Verification items for the finished model (mm, model axes). Face numbers are marked on the shaded views. Round coordinates to 2 decimals unless told otherwise and drop trailing zeros. Write each loop counter-clockwise with the first axis right and the second up, starting at its lowest first coordinate (ties: lowest second). Pieces come first, ordered by that corner, then holes.
from build123d import *

# Parameters (mm, degrees)
ESBO_O1_R                = 3
RESSALTO_EXTRUS_O1_DEPTH = 5
FILETE1_R                = 6
RESSALTO_EXTRUS_O2_DEPTH = 5
ESBO_O3_R                = 6
RESSALTO_EXTRUS_O3_DEPTH = 0.5


with BuildPart() as part:
    # Esboço1 → Ressalto-extrusão1 (new body)
    with BuildSketch(Plane.XY):
        Polygon((-8, -8), (-8, 8), (0, 8), (42.879830598, -10.223928004), (37.120169402, -23.776071996), (0, -8), align=None)
        Circle(ESBO_O1_R, mode=Mode.SUBTRACT)
    extrude(amount=RESSALTO_EXTRUS_O1_DEPTH)

    # Filete1
    filete1_edges = [part.edges().sort_by_distance(p)[0] for p in [
        (-8, -8, 2.5),
        (0, -8, 2.5),
        (37.120169402, -23.776071996, 2.5),
        (42.879830598, -10.223928004, 2.5),
        (0, 8, 2.5),
        (-8, 8, 2.5),
    ]]
    fillet(filete1_edges, radius=FILETE1_R)

    # Esboço2 → Ressalto-extrusão2 (add)
    with BuildSketch(Plane.XY.offset(5)):
        with BuildLine():
            Line((39.467013244, -18.254086485), (40.532986756, -15.745913515))
            ThreePointArc((40.532986756, -15.745913515), (40.575103841, -11.153905468), (37.357845087, -7.877084162))
            ThreePointArc((37.357845087, -7.877084162), (36.552086472, -7.588681558), (35.718304651, -7.395728495))
            ThreePointArc((35.718304651, -7.395728495), (27.413539889, -12.579084175), (31.598183891, -21.429228154))
            ThreePointArc((31.598183891, -21.429228154), (36.190191938, -21.471345238), (39.467013244, -18.254086485))
        make_face()
    extrude(amount=RESSALTO_EXTRUS_O2_DEPTH)

    # Esboço3 → Ressalto-extrusão3 (add)
    with BuildSketch(Plane.XY.offset(10)):
        with Locations((34.478014489, -14.653156158)):
            Circle(ESBO_O3_R)
    extrude(amount=RESSALTO_EXTRUS_O3_DEPTH)


solid = part.part
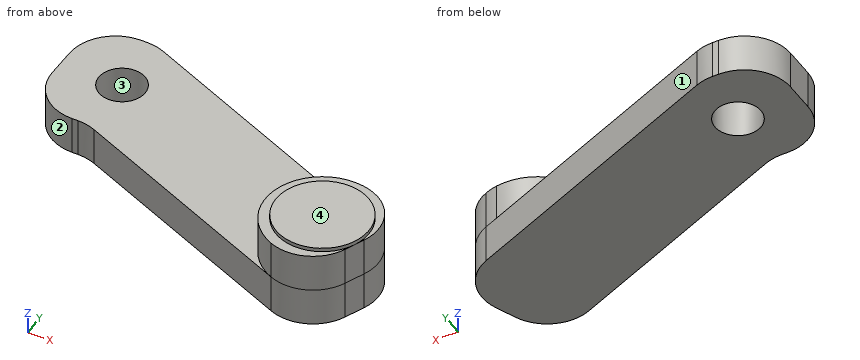
Q1. Sectioned sample at A-A (z = 0.5). Enter the section's corners in (x, y).
Recorded:
outline: (-8, -2) arc R6 ccw to (-2, -8) - (-1.22, -8) arc R6 cw to (1.12, -8.48) - (31.6, -21.43) arc R6 ccw to (39.47, -18.25) - (40.53, -15.75) arc R6 ccw to (37.36, -7.88) - (1.12, 7.52) arc R6 ccw to (-1.22, 8) - (-2, 8) arc R6 ccw to (-8, 2) - close; hole circle Ø6 at (0, 0)
Q2. Release check for a two-part mould opening along X. For the marked faces 1, 2, 3 and 4 record: released by +X, released by -X, zero draft, split by the parting line, or undercut.
Recorded:
face 1: released by +X
face 2: released by -X
face 3: undercut
face 4: zero draft
Q3. Depth check by flat-ended pin: P1, Ø1.5, axis at x = 4.5, y = -0.5, coming from the -Z side; P2, Ø1, axis at x = 34.5, z = 8, coming from the +Y side; P3, Ø9, axis at x = 7, y = -9, coming from the +Z side; P4, Ø1.5, axis at x = 33.5, z = 1, coming from the +Y side. Enter the tip coordinate at first touch or a pass-through.
Recorded:
P1: stops at z = 0
P2: stops at y = -7.29
P3: stops at z = 5
P4: stops at y = -5.92
Q4. Material ranges on line 1 along Y through (x, z) = (0, 3.65); line 2 along X through (y, z) = (1.75, 2.5); line 3 along Z through (x, y) = (13.5, -11.25), recorded low to high.
Recorded:
line 1: y = -8.13 to -3, 3 to 7.87
line 2: x = -8 to -2.44, 2.44 to 14.71
line 3: z = 0 to 5
Q5. Sectioned sample at C-C (y = 0). Enter the section's corners in (x, z), plus the area to 3 significant figures.
Recorded:
outline: (-8, 0) - (-3, 0) - (-3, 5) - (-8, 5) - close; (3, 0) - (18.82, 0) - (18.82, 5) - (3, 5) - close
area: 104 mm2
Q6. Sectioned sample at D-D (z = 7.25). Enter the section's corners in (x, y).
Recorded:
outline: (31.6, -21.43) arc R6 ccw to (39.47, -18.25) - (40.53, -15.75) arc R6 ccw to (37.36, -7.88) arc R7.36 ccw to start
Q7. Sectioned sample at B-B (x = 0). Enter the section's corners in (y, z).
Recorded:
outline: (-8.13, 0) - (-3, 0) - (-3, 5) - (-8.13, 5) - close; (3, 0) - (7.87, 0) - (7.87, 5) - (3, 5) - close
